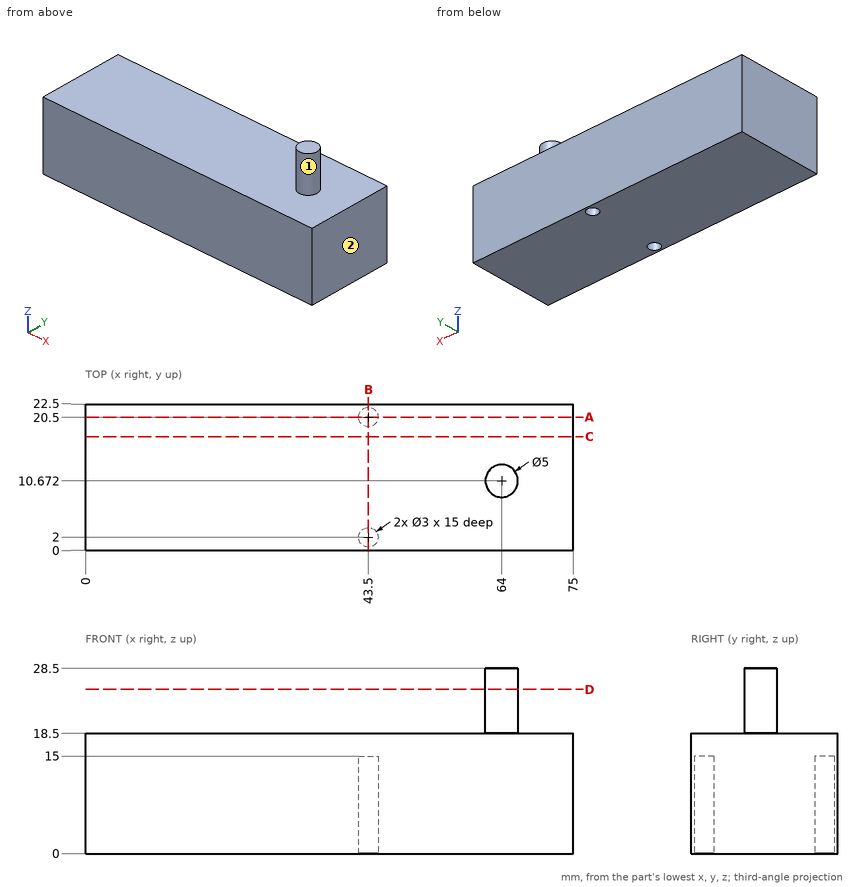
The drawing under review shows one solid part. Ordinate dimensions are in mm from its lowest x, y, z. A direction names the side the tool comes from. Give positions to 0.01 mm unless a question says otherwise; leave off trailing zeros. Order: outer loops, then holes, each group sorted by start corner. A loop starts at its lowest first (then second) coordinate and runs counter-clockwise, first axis right, second up. Notation, with made-up numbers: M -18.5,31 L -12.5,31 A6 cw -12.5,38 Z; hole C 7,45 d4. An arc over 180 degrees is marked long. Answer in a Markdown table with one row per item. Add a question column.
1. To check wall thickness, follow line 1 along Y through (x, z) = (43.5, 8); line 2 along Z through (x, y) = (35, 6.5); line 3 along X through (y, z) = (9, 22). State the ranges of each line that lie inside material, in increasing order.
2. Add section C-C on y = 17.5. State the section outline as (x, z) points, plus the area to 3 significant figures.
3. Add section D-D on z = 25.25. State the section outline as (x, y) points.
4. For pin 1 Ø3 at (x, z) = (65, 22) entering from +Y; pin 2 Ø2.5 at (x, y) = (43.5, 2) entering from +Z, all flat-tipped, find the tip position at first contact; note any pin that passes through.
5. Machinability: for the marked faces 1 and 2, which of the approach directions +Z, -Z, +X, -X, +Y, -Y give a long, thin tool a straight path to every point of the face, cutting with its end or side? Answer none if there is none.
6. Add section B-B on x = 43.5. State the section outline as (y, z) points.
7. Add section A-A on y = 20.5. State the section outline as (x, z) points, plus the area to 3 significant figures.
The answers:
| question | item | result |
|---|---|---|
| 1 | line 1 | 0 to 0.5, 3.5 to 19, 22 to 22.5 |
| 1 | line 2 | 0 to 18.5 |
| 1 | line 3 | 62.14 to 65.86 |
| 2 | outline | M 0,0 L 75,0 L 75,18.5 L 0,18.5 Z |
| 2 | area | 1,390 mm2 |
| 3 | outline | C 64,10.67 d5 |
| 4 | pin 1 | y = 13.17 |
| 4 | pin 2 | z = 18.5 |
| 5 | face 1 | +Z |
| 5 | face 2 | +Z, -Z, +X, +Y, -Y |
| 6 | outline | M 0,0 L 0.5,0 L 0.5,15 L 3.5,15 L 3.5,0 L 19,0 L 19,15 L 22,15 L 22,0 L 22.5,0 L 22.5,18.5 L 0,18.5 Z |
| 7 | outline | M 0,0 L 42,0 L 42,15 L 45,15 L 45,0 L 75,0 L 75,18.5 L 0,18.5 Z |
| 7 | area | 1,340 mm2 |
